CAD build for the part. Positions are in the model's coordinates, mm. A direction names the side the tool comes from. Round coordinates to 2 decimals unless told otherwise and drop trailing zeros. Write each loop counter-clockwise with the first axis right and the second up, starting at its lowest first coordinate (ties: lowest second). Pieces come first, ordered by that corner, then holes. Notation, with made-up numbers: (11.5, 58.5) - (19.5, 58.5) arc R22 ccw to (19.5, 66.5) - close; hole circle Ø1 at (-17, -28). An arc over 180 degrees is marked (long way). Answer in a Markdown table with one row per item.
```python
from build123d import *

# Parameters (mm, degrees)
CROQUIS1_R                   = 19.5
CROQUIS1_R_2                 = 16.6
SALIENTE_EXTRUIR1_DEPTH      = 60
SALIENTE_EXTRUIR3_DEPTH      = 35
SALIENTE_EXTRUIR3_DEPTH_BACK = 35
CROQUIS2_R                   = 19.5
CROQUIS2_R_2                 = 16.6
SALIENTE_EXTRUIR4_DEPTH      = 35
SALIENTE_EXTRUIR4_DEPTH_BACK = 35
CROQUIS3_R                   = 19.5
CROQUIS3_R_2                 = 16.6
CORTAR_EXTRUIR1_DEPTH        = 35
CORTAR_EXTRUIR1_DEPTH_BACK   = 35
CROQUIS5_R                   = 16.6
CORTAR_EXTRUIR2_DEPTH        = 35
CORTAR_EXTRUIR2_DEPTH_BACK   = 35
CROQUIS6_R                   = 16.6
CROQUIS7_R                   = 16.6
CORTAR_EXTRUIR3_DEPTH        = 60


with BuildPart() as part:
    # Croquis1 → Saliente-Extruir1 (new body)
    with BuildSketch(Plane(origin=(0, 0, 0), x_dir=(1, 0, 0), z_dir=(0, 1, 0))):
        with Locations(Location((0, 0, 0), (0, 0, 270))):
            Circle(CROQUIS1_R)
        with Locations(Location((0, 0, 0), (0, 0, 270))):
            Circle(CROQUIS1_R_2, mode=Mode.SUBTRACT)
    extrude(amount=SALIENTE_EXTRUIR1_DEPTH)

    # Croquis2 → Saliente-Extruir3 (add, two sides: drawn at the far end of the back side and taken through both)
    with BuildSketch(Plane(origin=(0, 0, 0), x_dir=(0, 0, -1), z_dir=(1, 0, 0)).offset(-SALIENTE_EXTRUIR3_DEPTH_BACK)):
        with Locations((0, 30)):
            Circle(CROQUIS2_R)
        with Locations((0, 30)):
            Circle(CROQUIS2_R_2, mode=Mode.SUBTRACT)
    extrude(amount=SALIENTE_EXTRUIR3_DEPTH + SALIENTE_EXTRUIR3_DEPTH_BACK)

    # Croquis3 → Saliente-Extruir4 (add, two sides: drawn at the far end of the back side and taken through both)
    with BuildSketch(Plane.XY.offset(-SALIENTE_EXTRUIR4_DEPTH_BACK)):
        with Locations((0, 30)):
            Circle(CROQUIS3_R)
        with Locations((0, 30)):
            Circle(CROQUIS3_R_2, mode=Mode.SUBTRACT)
    extrude(amount=SALIENTE_EXTRUIR4_DEPTH + SALIENTE_EXTRUIR4_DEPTH_BACK)

    # Croquis5 → Cortar-Extruir1 (cut, two sides: drawn at the far end of the back side and taken through both)
    with BuildSketch(Plane(origin=(0, 0, 0), x_dir=(0, 0, -1), z_dir=(1, 0, 0)).offset(-CORTAR_EXTRUIR1_DEPTH_BACK)):
        with Locations((0, 30)):
            Circle(CROQUIS5_R)
    extrude(amount=CORTAR_EXTRUIR1_DEPTH + CORTAR_EXTRUIR1_DEPTH_BACK, mode=Mode.SUBTRACT)

    # Croquis6 → Cortar-Extruir2 (cut, two sides: drawn at the far end of the back side and taken through both)
    with BuildSketch(Plane.XY.offset(-CORTAR_EXTRUIR2_DEPTH_BACK)):
        with Locations((0, 30)):
            Circle(CROQUIS6_R)
    extrude(amount=CORTAR_EXTRUIR2_DEPTH + CORTAR_EXTRUIR2_DEPTH_BACK, mode=Mode.SUBTRACT)

    # Croquis7 → Cortar-Extruir3 (cut)
    with BuildSketch(Plane(origin=(0, 0, 0), x_dir=(1, 0, 0), z_dir=(0, 1, 0))):
        with Locations(Location((0, 0, 0), (0, 0, 135))):
            Circle(CROQUIS7_R)
    extrude(amount=CORTAR_EXTRUIR3_DEPTH, mode=Mode.SUBTRACT)


solid = part.part
```
Q1. 3-axis set-ups, long thin cutter, end or side, ignore diameter. For faces 1 (the cylindrical face through (13.18, 6.19, -14.37)), 2 (the cylindrical face through (0.86, 53.58, -19.48)), 3 (the cylindrical face through (-14.37, 43.18, -26.9)), 4 (the cylindrical face through (-26.9, 43.18, 14.37)), 5 (the cylindrical face through (26.6, 43.18, 14.37)): which of +Z, -Z, +X, -X, +Y, -Y reach the whole face in a straight line?
Computed:
| item | result |
|---|---|
| face 1 | -Y |
| face 2 | +Y |
| face 3 | -Z |
| face 4 | -X |
| face 5 | +X |
Q2. Flat gauge pins, fed straight in: pin 1 (1 mm diameter, centred on x = -23, z = -8, fed in from +Y); pin 2 (2 mm diameter, centred on x = 27.5, y = 27.5, fed in from -Z); pin 3 (1 mm diameter, centred on y = 49, z = -10, fed in from +X); pin 4 (10 mm diameter, centred on y = 46.5, z = 15.5, fed in from +X). Where does each tip first touch, or does it go through?
Computed:
| item | result |
|---|---|
| pin 1 | stops at y = 48 |
| pin 2 | stops at z = -19.44 |
| pin 3 | stops at x = 17.03 |
| pin 4 | stops at x = 35 |
Q3. Drill centre lines: line 1 (Z direction, x = 0, y = 3.75); line 2 (Y direction, x = 0, z = 17); line 3 (Y direction, x = -15, z = 28). Where is each one in solid material? Low to high.
Computed:
| item | result |
|---|---|
| line 1 | z = -19.5 to -16.6, 16.6 to 19.5 |
| line 2 | y = 0 to 13.4, 46.6 to 60 |
| line 3 | y = 17.54 to 22.89, 37.11 to 42.46 |
Q4. Saw through at A-A on z = 0. List the corners of the cut face in (x, y).
Computed:
| item | result |
|---|---|
| outline | (-35, 10.5) - (-19.5, 10.5) - (-19.5, 0) - (-16.6, 0) - (-16.6, 13.4) - (-35, 13.4) - close; (-35, 46.6) - (-16.6, 46.6) - (-16.6, 60) - (-19.5, 60) - (-19.5, 49.5) - (-35, 49.5) - close; (16.6, 0) - (19.5, 0) - (19.5, 10.5) - (35, 10.5) - (35, 13.4) - (16.6, 13.4) - close; (16.6, 46.6) - (35, 46.6) - (35, 49.5) - (19.5, 49.5) - (19.5, 60) - (16.6, 60) - close |
Q5. Saw through at C-C on x = 18.5. List the corners of the cut face in (y, z).
Computed:
| item | result |
|---|---|
| outline | (0, -6.16) - (11.5, -6.16) arc R19.5 ccw to (23.84, -18.5) - (23.84, -35) - (36.16, -35) - (36.16, -18.5) arc R19.5 ccw to (48.5, -6.16) - (60, -6.16) - (60, 6.16) - (48.5, 6.16) arc R19.5 ccw to (36.16, 18.5) - (36.16, 35) - (23.84, 35) - (23.84, 18.5) arc R19.5 ccw to (11.5, 6.16) - (0, 6.16) - close; hole circle Ø33.2 at (30, 0) |
Q6. Saw through at B-B on x = 0. List the corners of the cut face in (y, z).
Computed:
| item | result |
|---|---|
| outline | (0, -19.5) - (10.5, -19.5) - (10.5, -35) - (13.4, -35) - (13.4, -16.6) - (0, -16.6) - close; (0, 16.6) - (13.4, 16.6) - (13.4, 35) - (10.5, 35) - (10.5, 19.5) - (0, 19.5) - close; (46.6, -35) - (49.5, -35) - (49.5, -19.5) - (60, -19.5) - (60, -16.6) - (46.6, -16.6) - close; (46.6, 16.6) - (60, 16.6) - (60, 19.5) - (49.5, 19.5) - (49.5, 35) - (46.6, 35) - close |
Q7. Saw through at D-D on y = 5.5. List the corners of the cut face in (x, z), then the cut area to 3 significant figures.
Computed:
| item | result |
|---|---|
| outline | circle Ø39 at (0, 0); hole circle Ø33.2 at (0, 0) |
| area | 329 mm2 |
